from build123d import *

# Parameters (mm, degrees)
BOSS_EXTRUDE1_DEPTH = 5
FILLET1_R           = 10
FILLET2_R           = 5
SKETCH2_R           = 1.65
CUT_EXTRUDE1_DEPTH  = 374.396572025
SKETCH3_R           = 1.65
CUT_EXTRUDE2_DEPTH  = 374.396572025
SKETCH4_R           = 1.65
CUT_EXTRUDE3_DEPTH  = 374.396572025
FILLET3_R           = 5


with BuildPart() as part:
    # Sketch1 → Boss-Extrude1 (new body)
    with BuildSketch(Plane(origin=(0, 0, 0), x_dir=(1, 0, 0), z_dir=(0, 1, 0))):
        Polygon((0, 0), (130, 0), (130, 12.5), (85, 12.5), (85, 103.5), (107.5, 103.5), (107.5, 246.5), (85, 246.5), (85, 337.5), (130, 337.5), (130, 350), (0, 350), (0, 337.5), (45, 337.5), (45, 246.5), (22.5, 246.5), (22.5, 103.5), (45, 103.5), (45, 12.5), (0, 12.5), align=None)
    extrude(amount=BOSS_EXTRUDE1_DEPTH)

    # Fillet1
    fillet1_edges = [part.edges().sort_by_distance(p)[0] for p in [
        (130, 2.5, 0),
        (0, 2.5, 0),
    ]]
    fillet(fillet1_edges, radius=FILLET1_R)

    # Fillet2
    fillet2_edges = [part.edges().sort_by_distance(p)[0] for p in [
        (22.5, 2.5, -103.5),
        (22.5, 2.5, -246.5),
        (0, 2.5, -350),
        (130, 2.5, -350),
        (107.5, 2.5, -246.5),
        (107.5, 2.5, -103.5),
    ]]
    fillet(fillet2_edges, radius=FILLET2_R)

    # Sketch2 → Cut-Extrude1 (cut, through all)
    with BuildSketch(Plane(origin=(0, 5, 0), x_dir=(1, 0, 0), z_dir=(0, 1, 0))):
        with Locations(Location((32.5, 240, 0), (0, 0, 270))):
            Circle(SKETCH2_R)
        with Locations(Location((32.5, 175, 0), (0, 0, 270))):
            Circle(SKETCH2_R)
        with Locations(Location((32.5, 110, 0), (0, 0, 270))):
            Circle(SKETCH2_R)
        with Locations(Location((97.5, 110, 0), (0, 0, 90))):
            Circle(SKETCH2_R)
        with Locations(Location((97.5, 175, 0), (0, 0, 90))):
            Circle(SKETCH2_R)
        with Locations(Location((97.5, 240, 0), (0, 0, 90))):
            Circle(SKETCH2_R)
    extrude(amount=-CUT_EXTRUDE1_DEPTH, mode=Mode.SUBTRACT)

    # Sketch3 → Cut-Extrude2 (cut, through all)
    with BuildSketch(Plane(origin=(0, 5, 0), x_dir=(1, 0, 0), z_dir=(0, 1, 0))):
        with Locations(Location((8.75, 8.75, 0), (0, 0, 270))):
            Circle(SKETCH3_R)
        with Locations(Location((121.25, 8.75, 0), (0, 0, 90))):
            Circle(SKETCH3_R)
    extrude(amount=-CUT_EXTRUDE2_DEPTH, mode=Mode.SUBTRACT)

    # Sketch4 → Cut-Extrude3 (cut, through all)
    with BuildSketch(Plane(origin=(0, 5, 0), x_dir=(1, 0, 0), z_dir=(0, 1, 0))):
        with Locations(Location((8.75, 341.25, 0), (0, 0, 270))):
            Circle(SKETCH4_R)
        with Locations(Location((121.25, 341.25, 0), (0, 0, 90))):
            Circle(SKETCH4_R)
    extrude(amount=-CUT_EXTRUDE3_DEPTH, mode=Mode.SUBTRACT)

    # Fillet3
    fillet3_edges = [part.edges().sort_by_distance(p)[0] for p in [
        (45, 2.5, -12.5),
        (45, 2.5, -103.5),
        (45, 2.5, -246.5),
        (45, 2.5, -337.5),
        (85, 2.5, -337.5),
        (85, 2.5, -246.5),
        (85, 2.5, -103.5),
        (85, 2.5, -12.5),
    ]]
    fillet(fillet3_edges, radius=FILLET3_R)


solid = part.part
The listing builds one solid part. Answer for the finished solid, in the listing's coordinates (mm). Coordinates: 2 decimals unless noted, no trailing zeros. Loops run counter-clockwise (first coordinate to the right, second up) from the corner with the lowest first, then second, coordinate; pieces in that order, holes last.
1) Find section D-D on z = -44. Write down the section's boundary in (x, y).
2) Find the intervals of material crossed by L1, parallel to X at y = 3.1, z = -175; L2, parallel to Z at x = 38, y = 1.6; L3, parallel to X at y = 1.5, z = -8.75, in increasing order.
3) Find section A-A on x = 110.5. Write down the section's boundary in (y, z), then the cut area to 3 significant figures.
4) Flat-ended cylindrical pins translate along their axes: pin 1 Ø1.5 at (y, z) = (2.5, -49) entering from -X; pin 2 Ø5.5 at (x, z) = (97.5, -110) entering from +Y; pin 3 Ø1.5 at (y, z) = (2.5, -96.5) entering from +X; pin 4 Ø2.5 at (y, z) = (2.5, -200.5) entering from -X. Find the tip coordinate at first contact, or state that the pin passes through.
5) Find section B-B on y = 3.1. Give the number of separate pieces and of enclosed holes in the cut face, then the cut area to 3 significant figures.
6) Find section C-C on z = -150.5. Write down the section's boundary in (x, y).
Values:
1. outline: (45, 0) - (85, 0) - (85, 5) - (45, 5) - close
2. L1: x = 22.5 to 30.85, 34.15 to 95.85, 99.15 to 107.5
2. L2: z = -350 to -337.5, -246.5 to -103.5, -12.5 to 0
2. L3: x = 0.08 to 7.1, 10.4 to 119.6, 122.9 to 129.92
3. outline: (0, -350) - (5, -350) - (5, -337.5) - (0, -337.5) - close; (0, -12.5) - (5, -12.5) - (5, 0) - (0, 0) - close
3. area: 125 mm2
4. pin 1: stops at x = 45
4. pin 2: stops at y = 5
4. pin 3: stops at x = 85
4. pin 4: stops at x = 22.5
5. separate pieces: 1
5. enclosed holes: 10
5. area: 22,600 mm2
6. outline: (22.5, 0) - (107.5, 0) - (107.5, 5) - (22.5, 5) - close
